Verification items for this drawing (mm, ordinates from the low corner). A direction names the side the tool comes from. Round coordinates to 2 decimals unless told otherwise and drop trailing zeros. Loops run counter-clockwise (first coordinate to the right, second up) from the corner with the lowest first, then second, coordinate; pieces in that order, holes last. Notation, with made-up numbers: M 9,47 L 41,47 A15 ccw 41,68 Z; hole C 23.5,-20.75 d10. An arc over 180 degrees is marked long. Write item = value, one per line. Start each with the question number.
(1) Cross-section at D-D on y = 34. Record the boundary of the cut face in (x, z), plus the area to 3 significant figures.
(2) Cross-section at A-A on z = 10. Record the boundary of the cut face in (x, y).
(3) Mould release check, pull along Z, two halves, no side actions. Record for the marked faces 1, 2, 3 and 4: pulls with the +Z half, pulls with the -Z half, needs draft (parallel to the pull), parting line crosses it, or undercut.
(4) Set-up check for the marked faces 5 and 6: record each of +Z, -Z, +X, -X, +Y, -Y from which the full face is reachable in a straight line by a thin tool's end or side.
(5) Cross-section at C-C on z = 29.5. Record the boundary of the cut face in (x, y).
(6) Go/stop test with flat-tipped pins: P1, Ø12, axis at x = 23, y = 33, coming from the -Z side; P2, Ø15, axis at y = 12, z = 10, coming from the +X side; P3, Ø11, axis at x = 36, y = 10.5, coming from the -Z side; P4, Ø5.5, axis at x = 46.5, z = 10, coming from the -Y side. Record where each tip stops, or that it passes through.
(7) Cross-section at B-B on x = 43.5. Record the boundary of the cut face in (y, z), plus the area to 3 significant figures.
(8) Scan lines: L1, parallel to X at y = 28.5, z = 13; L2, parallel to Z at x = 35, y = 31; L3, parallel to Z at x = 37.5, y = 28. Record each from-to range of solid material in increasing order. Write a range as from..to.
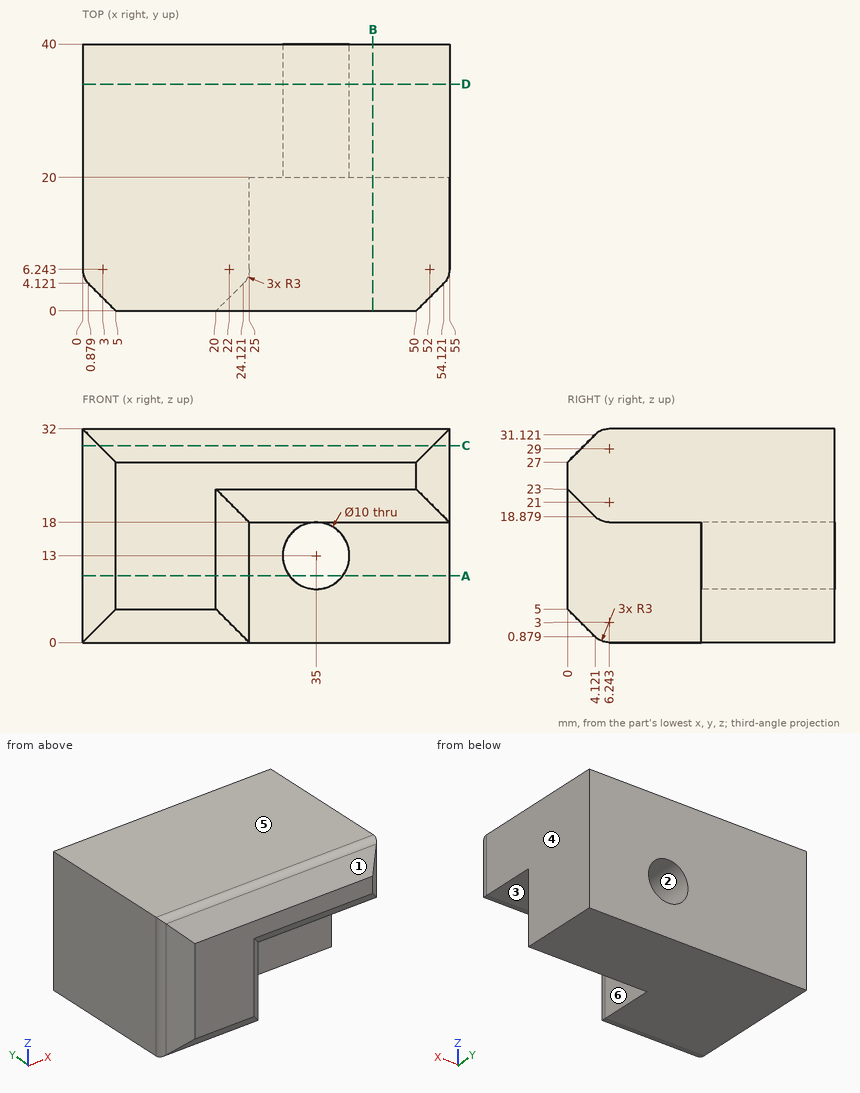
Result:
q1.outline = M 0,0 L 55,0 L 55,32 L 0,32 Z; hole C 35,13 d10
q1.area = 1,680 mm^2
q2.outline = M 0,6.24 A3 ccw 0.88,4.12 L 5,0 L 20,0 L 24.12,4.12 A3 ccw 25,6.24 L 25,20 L 31,20 L 31,40 L 0,40 Z; M 39,20 L 55,20 L 55,40 L 39,40 Z
q3.face_1 = pulls with the +Z half
q3.face_2 = undercut
q3.face_3 = pulls with the -Z half
q3.face_4 = needs draft
q4.face_5 = +Z, +X, -X, +Y, -Y
q4.face_6 = -Z, +X, -Y
q5.outline = M 0,6.24 A3 ccw 0.88,4.12 L 2.5,2.5 L 52.5,2.5 L 54.12,4.12 A3 ccw 55,6.24 L 55,40 L 0,40 Z
q6.P1 = 0
q6.P2 = 25
q6.P3 = 18
q6.P4 = 20
q7.outline = M 0,23 L 4.12,18.88 A3 ccw 6.24,18 L 20,18 L 20,0 L 40,0 L 40,32 L 6.24,32 A3 ccw 4.12,31.12 L 0,27 Z
q7.area = 895 mm^2
q8.L1 = 0..30, 40..55
q8.L2 = 0..8, 18..32
q8.L3 = 0..8.67, 17.33..32
